Could you check a few things on this model? Use its own coordinates, in mm. Coordinates: 2 decimals unless noted, no trailing zeros. Loops run counter-clockwise (first coordinate to the right, second up) from the corner with the lowest first, then second, coordinate; pieces in that order, holes last.
1) Imagine slicing it at B-B on x = 74.25. Please give me the cut outline in (y, z) (3 decimals), plus the area to 3 significant figures.
2) Imagine slicing it at A-A on z = -37.2. Please give me the cut outline in (x, y) (3 decimals).
3) If I drill on line 1 along X through (y, z) = (-3.95, -37.2) (3 decimals); line 2 along Z through (x, y) = (89.25, -3.5) (3 decimals); line 3 along Z through (x, y) = (10, -3.4) (3 decimals), over which ranges is the centre line in solid material (lowest first)?
4) Imagine slicing it at D-D on x = 84.5. Please give me the cut outline in (y, z) (3 decimals), plus the area to 3 significant figures.
5) Imagine slicing it at C-C on y = -3.95. Please give me the cut outline in (x, z) (3 decimals).
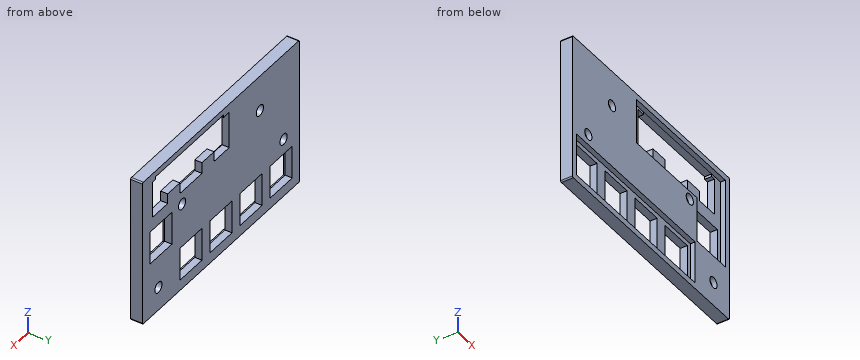
```python
from build123d import *

# Parameters (mm, degrees)
SKETCH1_W           = 99.3
SKETCH1_H           = 62.2
SKETCH1_R           = 2.275
SKETCH1_W_2         = 14
SKETCH1_H_2         = 14
BOSS_EXTRUDE1_DEPTH = 3
SKETCH6_W           = 99.3
SKETCH6_H           = 62.2
SKETCH6_W_2         = 75.15
SKETCH6_H_2         = 18
SKETCH6_R           = 2.275
BOSS_EXTRUDE2_DEPTH = 2
FILLET1_R           = 0.5


with BuildPart() as part:
    # Sketch1 → Boss-Extrude1 (new body)
    with BuildSketch(Plane(origin=(0, 0, 0), x_dir=(1, 0, 0), z_dir=(0, 1, 0))):
        with Locations((49.65, 31.1)):
            Rectangle(SKETCH1_W, SKETCH1_H)
        with Locations(Location((10, 37.2, 0), (0, 0, 270))):
            Circle(SKETCH1_R, mode=Mode.SUBTRACT)
        with Locations(Location((89.25, 52.2, 0), (0, 0, 270))):
            Circle(SKETCH1_R, mode=Mode.SUBTRACT)
        with Locations(Location((74.25, 25.05, 0), (0, 0, 270))):
            Circle(SKETCH1_R, mode=Mode.SUBTRACT)
        with Locations(Location((25, 15.05, 0), (0, 0, 270))):
            Circle(SKETCH1_R, mode=Mode.SUBTRACT)
        with Locations((11.525, 50.675)):
            Rectangle(SKETCH1_W_2, SKETCH1_H_2, mode=Mode.SUBTRACT)
        with Locations((30.575, 50.675)):
            Rectangle(SKETCH1_W_2, SKETCH1_H_2, mode=Mode.SUBTRACT)
        with Locations((49.625, 50.675)):
            Rectangle(SKETCH1_W_2, SKETCH1_H_2, mode=Mode.SUBTRACT)
        with Locations((68.675, 50.675)):
            Rectangle(SKETCH1_W_2, SKETCH1_H_2, mode=Mode.SUBTRACT)
        with Locations((87.725, 31.625)):
            Rectangle(SKETCH1_W_2, SKETCH1_H_2, mode=Mode.SUBTRACT)
        Polygon((61.675, 19.575), (75.675, 19.575), (75.675, 14.875), (83.35, 14.875), (83.35, 19.105), (92.925, 19.105), (92.925, 3.605), (91.1, 3.605), (91.1, 2.5), (47.975, 2.5), (47.975, 3.605), (44.425, 3.605), (44.425, 19.105), (54, 19.105), (54, 14.875), (61.675, 14.875), align=None, mode=Mode.SUBTRACT)
    extrude(amount=-BOSS_EXTRUDE1_DEPTH)

    # Sketch6 → Boss-Extrude2 (add)
    with BuildSketch(Plane.XZ.offset(3)):
        with Locations((49.65, -31.1)):
            Rectangle(SKETCH6_W, SKETCH6_H)
        with Locations((40.1, -50.675)):
            Rectangle(SKETCH6_W_2, SKETCH6_H_2, mode=Mode.SUBTRACT)
        with Locations(Location((10, -37.2, 0), (0, 0, 90))):
            Circle(SKETCH6_R, mode=Mode.SUBTRACT)
        with Locations(Location((89.25, -52.2, 0), (0, 0, 90))):
            Circle(SKETCH6_R, mode=Mode.SUBTRACT)
        with Locations(Location((25, -15.05, 0), (0, 0, 90))):
            Circle(SKETCH6_R, mode=Mode.SUBTRACT)
        with Locations(Location((74.25, -25.05, 0), (0, 0, 90))):
            Circle(SKETCH6_R, mode=Mode.SUBTRACT)
        Polygon((96.725, -2.5), (96.725, -40.562928412), (78.725, -40.562928412), (78.725, -21.575), (40.625, -21.575), (40.625, -2.5), (47.975, -2.5), (91.1, -2.5), align=None, mode=Mode.SUBTRACT)
    extrude(amount=BOSS_EXTRUDE2_DEPTH)

    # Fillet1
    fillet1_edges = [part.edges().sort_by_distance(p)[0] for p in [
        (0, -2.5, 0),
        (0, -2.5, -62.2),
        (99.3, -2.5, -62.2),
        (99.3, -2.5, 0),
    ]]
    fillet(fillet1_edges, radius=FILLET1_R)


solid = part.part
```
Filled in:
1. outline: (-5, -62.2) - (0, -62.2) - (0, -57.675) - (-3, -57.675) - (-3, -59.675) - (-5, -59.675) - close; (-5, -41.675) - (-3, -41.675) - (-3, -43.675) - (0, -43.675) - (0, -27.325) - (-5, -27.325) - close; (-5, -22.775) - (0, -22.775) - (0, -19.575) - (-3, -19.575) - (-3, -21.575) - (-5, -21.575) - close; (-5, -2.5) - (0, -2.5) - (0, 0) - (-5, 0) - close
1. area: 121 mm2
2. outline: (0, -5) - (7.725, -5) - (7.725, 0) - (0, 0) - close; (12.275, -5) - (78.725, -5) - (78.725, -3) - (80.725, -3) - (80.725, 0) - (12.275, 0) - close; (94.725, -3) - (96.725, -3) - (96.725, -5) - (99.3, -5) - (99.3, 0) - (94.725, 0) - close
3. line 1: x = 0 to 7.725, 12.275 to 78.725, 96.725 to 99.3
3. line 2: z = -62.2 to -54.475, -49.925 to -40.563, -2.5 to 0
3. line 3: z = -62.2 to -59.675, -41.675 to -39.475, -34.925 to 0
4. outline: (-5, -62.2) - (0, -62.2) - (0, -38.625) - (-3, -38.625) - (-3, -40.563) - (-5, -40.563) - close; (-5, -2.5) - (0, -2.5) - (0, 0) - (-5, 0) - close; (-3, -24.625) - (0, -24.625) - (0, -19.105) - (-3, -19.105) - close
4. area: 143 mm2
5. outline: (0, -61.7) arc R0.5 ccw to (0.5, -62.2) - (98.8, -62.2) arc R0.5 ccw to (99.3, -61.7) - (99.3, -0.5) arc R0.5 ccw to (98.8, 0) - (0.5, 0) arc R0.5 ccw to (0, -0.5) - close; hole (2.525, -59.675) - (77.675, -59.675) - (77.675, -41.675) - (2.525, -41.675) - close; hole circle Ø4.55 at (10, -37.2); hole circle Ø4.55 at (25, -15.05); hole (40.625, -21.575) - (78.725, -21.575) - (78.725, -40.563) - (96.725, -40.563) - (96.725, -2.5) - (40.625, -2.5) - close; hole circle Ø4.55 at (74.25, -25.05); hole circle Ø4.55 at (89.25, -52.2)
